from build123d import *

# Parameters (mm, degrees)
SKETCH1_W           = 32.2
SKETCH1_H           = 26.6
SKETCH1_W_2         = 23
SKETCH1_H_2         = 12.9
SKETCH1_W_3         = 7.5
BOSS_EXTRUDE1_DEPTH = 4.25
SKETCH1_3_W         = 32.2
SKETCH1_3_H         = 26.6
SKETCH1_3_W_2       = 23
SKETCH1_3_H_2       = 12.9
BOSS_EXTRUDE2_DEPTH = 3.7
SKETCH2_R           = 1.025
CUT_EXTRUDE1_DEPTH  = 5
SKETCH3_W           = 32.2
SKETCH3_H           = 3.7
SKETCH3_H_2         = 10
BOSS_EXTRUDE3_DEPTH = 18.3
SKETCH4_W           = 4.6
SKETCH4_H           = 3.7
BOSS_EXTRUDE4_DEPTH = 12.7
CUT_EXTRUDE2_REACH  = 28.6
SKETCH5_R           = 1


with BuildPart() as part:
    # Sketch1 → Boss-Extrude1 (new body)
    with BuildSketch(Plane(origin=(0, 0, 0), x_dir=(1, 0, 0), z_dir=(0, 1, 0))):
        with Locations((-5.05, 3.15)):
            Rectangle(SKETCH1_W, SKETCH1_H)
        with Locations((-5.05, 0)):
            Rectangle(SKETCH1_W_2, SKETCH1_H_2, mode=Mode.SUBTRACT)
        with Locations((-12.8, 0)):
            Rectangle(SKETCH1_W_3, SKETCH1_H_2)
    extrude(amount=-BOSS_EXTRUDE1_DEPTH)

    # Sketch1_3 → Boss-Extrude2 (add)
    with BuildSketch(Plane(origin=(0, 0, 0), x_dir=(1, 0, 0), z_dir=(0, 1, 0))):
        with Locations((-5.05, 3.15)):
            Rectangle(SKETCH1_3_W, SKETCH1_3_H)
        with Locations((-5.05, 0)):
            Rectangle(SKETCH1_3_W_2, SKETCH1_3_H_2, mode=Mode.SUBTRACT)
    extrude(amount=BOSS_EXTRUDE2_DEPTH)

    # Sketch2 → Cut-Extrude1 (cut)
    with BuildSketch(Plane(origin=(0, 3.7, 0), x_dir=(1, 0, 0), z_dir=(0, 1, 0))):
        with Locations((-18.75, 0)):
            Circle(SKETCH2_R)
        with Locations((8.65, 0)):
            Circle(SKETCH2_R)
    extrude(amount=-CUT_EXTRUDE1_DEPTH, mode=Mode.SUBTRACT)

    # Sketch3 → Boss-Extrude3 (add)
    with BuildSketch(Plane(origin=(0, 3.7, 0), x_dir=(1, 0, 0), z_dir=(0, 1, 0))):
        with Locations((-5.05, -8.3)):
            Rectangle(SKETCH3_W, SKETCH3_H)
        with Locations((-5.05, 11.45)):
            Rectangle(SKETCH3_W, SKETCH3_H_2)
    extrude(amount=BOSS_EXTRUDE3_DEPTH)

    # Sketch4 → Boss-Extrude4 (add)
    with BuildSketch(Plane(origin=(0, 22, 0), x_dir=(1, 0, 0), z_dir=(0, 1, 0))):
        Polygon((-21.15, 16.45), (-16.55, 16.45), (6.45, 16.45), (11.05, 16.45), (11.05, 7.55), (6.45, 7.55), (6.45, 11.85), (-16.55, 11.85), (-16.55, 6.45), (-21.15, 6.45), align=None)
        with Locations((-18.85, -8.3)):
            Rectangle(SKETCH4_W, SKETCH4_H)
        with Locations((8.75, -8.3)):
            Rectangle(SKETCH4_W, SKETCH4_H)
    extrude(amount=BOSS_EXTRUDE4_DEPTH)

    # Sketch5 → Cut-Extrude2 (cut, up to next)
    with BuildSketch(Plane.XY.offset(10.15), mode=Mode.PRIVATE) as cut_extrude2_sk1:
        with Locations((-18.85, 28.35)):
            Circle(SKETCH5_R)
    cut_extrude2_tool1 = extrude(cut_extrude2_sk1.sketch, amount=-CUT_EXTRUDE2_REACH, mode=Mode.PRIVATE) & part.part
    add(cut_extrude2_tool1.solids().sort_by_distance((-18.85, 28.35, 10.15))[0], mode=Mode.SUBTRACT)
    # Sketch5 → Cut-Extrude2 (cut, up to next)
    with BuildSketch(Plane.XY.offset(10.15), mode=Mode.PRIVATE) as cut_extrude2_sk2:
        with Locations((8.75, 28.35)):
            Circle(SKETCH5_R)
    cut_extrude2_tool2 = extrude(cut_extrude2_sk2.sketch, amount=-CUT_EXTRUDE2_REACH, mode=Mode.PRIVATE) & part.part
    add(cut_extrude2_tool2.solids().sort_by_distance((8.75, 28.35, 10.15))[0], mode=Mode.SUBTRACT)


solid = part.part
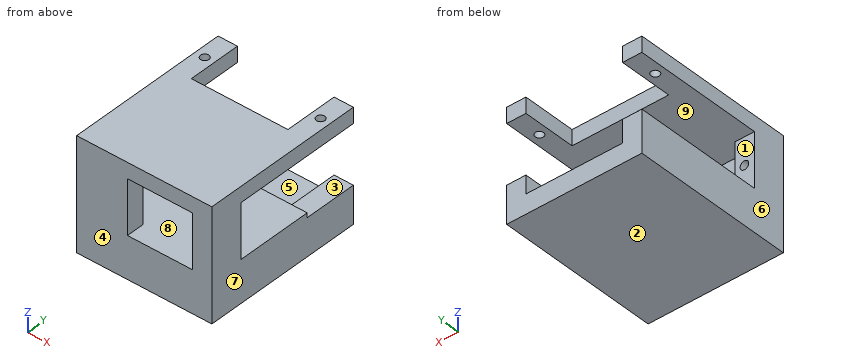
Model file for the job. Use its own axes, mm. Face numbers are marked on the shaded views. A direction names the side the tool comes from. Coordinates: 2 decimals unless noted, no trailing zeros. Write each loop counter-clockwise with the first axis right and the second up, starting at its lowest first coordinate (ties: lowest second). Pieces come first, ordered by that corner, then holes. Notation, with made-up numbers: (0.5, 86) -> (38.5, 86) arc R14 ccw to (38.5, 92) -> close; hole circle Ø11 at (19.25, -7.5). An arc over 180 degrees is marked (long way). One line per item, written item: value. Start each with the question number.
1) Slice it at B-B on x = 0. Write the cut outline in (y, z), then the cut area to 3 significant figures.
2) Slice it at D-D on x = -10. Write the cut outline in (y, z), then the cut area to 3 significant figures.
3) Flat gauge pins, fed straight in: pin 1 Ø4 at (x, z) = (-3.5, 8.5) entering from +Y; pin 2 Ø4 at (x, z) = (-13, 2) entering from +Y; pin 3 Ø6 at (x, y) = (-11, 23) entering from +Z; pin 4 Ø1.2 at (x, y) = (8.75, 28.35) entering from +Z. Where does each tip first touch, or does it go through?
4) Pull direction X, two halves, no side cores. Call the marked faces 6, 7, 8 and 9: +X half, -X half, draft (parallel to the pull), parting line (faces both ways), or undercut.
5) Which spindle directions (+Z, -Z, +X, -X, +Y, -Y) get a long thin tool onto all of the face, cutting with end or side? Do the marked faces 1, 2, 3, 4 and 5. Say none if no direction does.
6) Slice it at C-C on y = 4.5. Write the cut outline in (x, z).
7) Probe probe 1 along Z at (x, y) = (-15, 17); probe 2 along Y at (x, z) = (8.75, 8.25); probe 3 along X at (y, z) = (2, 0) (3 decimals). List the from-to ranges inside material, lowest first.
8) Slice it at A-A on y = 28.35. Write the cut outline in (x, z).
Answers follow:
1. outline: (-4.25, -16.45) -> (34.7, -16.45) -> (34.7, -11.85) -> (22, -11.85) -> (22, -6.45) -> (-4.25, -6.45) -> close; (-4.25, 6.45) -> (22, 6.45) -> (22, 10.15) -> (-4.25, 10.15) -> close
1. area: 418 mm2
2. outline: (-4.25, -16.45) -> (34.7, -16.45) -> (34.7, -11.85) -> (22, -11.85) -> (22, -6.45) -> (0, -6.45) -> (0, 6.45) -> (22, 6.45) -> (22, 10.15) -> (-4.25, 10.15) -> close
2. area: 473 mm2
3. pin 1: y = 22
3. pin 2: y = 0
3. pin 3: z = 10.15
3. pin 4: z = -7.55
4. face 6: -X half
4. face 7: +X half
4. face 8: undercut
4. face 9: undercut
5. face 1: +X, -X, +Y
5. face 2: -Z, +X, -X, +Y, -Y
5. face 3: +X, +Y
5. face 4: +Z, -Z, +X, -X, -Y
5. face 5: +Z, +Y
6. outline: (-21.15, -16.45) -> (11.05, -16.45) -> (11.05, -6.45) -> (-21.15, -6.45) -> close; (-21.15, 6.45) -> (11.05, 6.45) -> (11.05, 10.15) -> (-21.15, 10.15) -> close
7. probe 1: -16.45 to -6.45, 6.45 to 10.15
7. probe 2: -4.25 to 27.35, 29.35 to 34.7
7. probe 3: -21.15 to -19.775, -17.725 to -16.55, 6.45 to 7.625, 9.675 to 11.05
8. outline: (-21.15, -16.45) -> (11.05, -16.45) -> (11.05, -7.55) -> (6.45, -7.55) -> (6.45, -11.85) -> (-16.55, -11.85) -> (-16.55, -6.45) -> (-21.15, -6.45) -> close; (-21.15, 6.45) -> (-19.85, 6.45) -> (-19.85, 10.15) -> (-21.15, 10.15) -> close; (-17.85, 6.45) -> (-16.55, 6.45) -> (-16.55, 10.15) -> (-17.85, 10.15) -> close; (6.45, 6.45) -> (7.75, 6.45) -> (7.75, 10.15) -> (6.45, 10.15) -> close; (9.75, 6.45) -> (11.05, 6.45) -> (11.05, 10.15) -> (9.75, 10.15) -> close
